Verification items for the finished model (mm, model axes). Coordinates: 2 decimals unless noted, no trailing zeros. Order: outer loops, then holes, each group sorted by start corner. A loop starts at its lowest first (then second) coordinate and runs counter-clockwise, first axis right, second up. Notation, with made-up numbers: (89.25, 8) - (143.25, 8) arc R6 ccw to (143.25, 15) - close; hole circle Ø9 at (31, 63). An arc over 180 degrees is marked (long way). One line per question, with ' | ' between items. Start each with the question number.
from build123d import *

# Parameters (mm, degrees)
F0_R     = 3.3
F0_R_2   = 4.5
F1_DEPTH = 1
F2_D     = 6.6
F3_D     = 6.6
F4_D     = 9


with BuildPart() as f1:
    # F0 (on Top) → F1 (new body)
    with BuildSketch(Plane.XY):
        with Locations((0, 16)):
            Circle(F0_R)
        Circle(F0_R_2)
        with Locations((0, -16)):
            Circle(F0_R)
        with BuildLine():
            ThreePointArc((0, 10), (6.123724, 7.905694), (9.682458, 2.5))
            Line((9.682458, 2.5), (5.809475, 17.5))
            ThreePointArc((5.809475, 17.5), (5.952178, 16.756026), (6, 16))
            ThreePointArc((6, 16), (4.242641, 11.757359), (0, 10))
        make_face()
        with BuildLine():
            ThreePointArc((-9.682458, 2.5), (-6.123724, 7.905694), (0, 10))
            ThreePointArc((0, 10), (-4.743416, 12.325765), (-5.809475, 17.5))
            Line((-5.809475, 17.5), (-9.682458, 2.5))
        make_face()
        with BuildLine():
            Line((5.809475, -17.5), (9.682458, -2.5))
            ThreePointArc((9.682458, -2.5), (6.123724, -7.905694), (0, -10))
            ThreePointArc((0, -10), (4.242641, -11.757359), (6, -16))
            ThreePointArc((6, -16), (5.952178, -16.756026), (5.809475, -17.5))
        make_face()
        with BuildLine():
            ThreePointArc((-5.809475, -17.5), (-4.743416, -12.325765), (0, -10))
            ThreePointArc((0, -10), (-6.123724, -7.905694), (-9.682458, -2.5))
            Line((-9.682458, -2.5), (-5.809475, -17.5))
        make_face()
        with BuildLine():
            ThreePointArc((6, -16), (4.242641, -11.757359), (0, -10))
            ThreePointArc((0, -10), (-4.743416, -12.325765), (-5.809475, -17.5))
            ThreePointArc((-5.809475, -17.5), (0, -22), (5.809475, -17.5))
            ThreePointArc((5.809475, -17.5), (5.952178, -16.756026), (6, -16))
        make_face()
        with Locations((0, -16)):
            Circle(F0_R, mode=Mode.SUBTRACT)
        with BuildLine():
            ThreePointArc((-5.809475, 17.5), (-4.743416, 12.325765), (0, 10))
            ThreePointArc((0, 10), (4.242641, 11.757359), (6, 16))
            ThreePointArc((6, 16), (5.952178, 16.756026), (5.809475, 17.5))
            ThreePointArc((5.809475, 17.5), (0, 22), (-5.809475, 17.5))
        make_face()
        with Locations((0, 16)):
            Circle(F0_R, mode=Mode.SUBTRACT)
        with BuildLine():
            ThreePointArc((9.682458, -2.5), (9.920297, -1.260043), (10, 0))
            ThreePointArc((10, 0), (9.920297, 1.260043), (9.682458, 2.5))
            ThreePointArc((9.682458, 2.5), (6.123724, 7.905694), (0, 10))
            ThreePointArc((0, 10), (-6.123724, 7.905694), (-9.682458, 2.5))
            ThreePointArc((-9.682458, 2.5), (-10, 0), (-9.682458, -2.5))
            ThreePointArc((-9.682458, -2.5), (-6.123724, -7.905694), (0, -10))
            ThreePointArc((0, -10), (6.123724, -7.905694), (9.682458, -2.5))
        make_face()
        Circle(F0_R_2, mode=Mode.SUBTRACT)
    extrude(amount=F1_DEPTH)

    # F2 (through all)
    with Locations(Plane(origin=(0, 0, 0), x_dir=(1, 0, 0), z_dir=(0, 0, -1))):
        with Locations((0, 16)):
            Hole(F2_D / 2)

    # F3 (through all)
    with Locations(Plane(origin=(0, 0, 0), x_dir=(1, 0, 0), z_dir=(0, 0, -1))):
        with Locations((0, -16)):
            Hole(F3_D / 2)

    # F4 (through all)
    with Locations(Plane(origin=(0, 0, 0), x_dir=(1, 0, 0), z_dir=(0, 0, -1))):
        with Locations((0, 0)):
            Hole(F4_D / 2)


solid = f1.part
Item 1: Section check D-D (x = 4). Record the cut outline in (y, z).
Item 2: Section check B-B (x = 0). Record the cut outline in (y, z).
Item 3: Section check A-A (z = 0.3). Record the cut outline in (x, y).
Item 4: Mould release check, pull along X, two halves, no side actions. Record for faces 1 (the flat face through (7.72, -10.1, 0.49)), 2 (the cylindrical face through (-10, 0, 0.5)), 3 (the cylindrical face through (-2.619, -18.008, 0.493)), 4 (the cylindrical face through (-2.43, 18.23, 0.49)): +X half, -X half, draft (parallel to the pull), parting line (faces both ways), or undercut.
Item 5: Thickness scan on probe 1 along Y at (x, z) = (1.5, 0.2); probe 2 along Y at (x, z) = (-2, 0.8); probe 3 along X at (y, z) = (-1, 0.7). Record the ranges inside material, lowest first. Write a range as from..to.
Item 6: Gauge pin test, flat end, axial feed: pin 1 (2 mm diameter, centred on x = 0, y = 2, fed in from -Z). Record the tip position at first contact, or that the pin passes through.
Item 7: Section check C-C (y = -16). Record the cut outline in (x, z).
Completed:
1) outline: (-20.47, 0) - (-2.06, 0) - (-2.06, 1) - (-20.47, 1) - close; (2.06, 0) - (20.47, 0) - (20.47, 1) - (2.06, 1) - close
2) outline: (-22, 0) - (-19.3, 0) - (-19.3, 1) - (-22, 1) - close; (-12.7, 0) - (-4.5, 0) - (-4.5, 1) - (-12.7, 1) - close; (4.5, 0) - (12.7, 0) - (12.7, 1) - (4.5, 1) - close; (19.3, 0) - (22, 0) - (22, 1) - (19.3, 1) - close
3) outline: (-9.68, -2.5) - (-5.81, -17.5) arc R6 ccw to (5.81, -17.5) - (9.68, -2.5) arc R10 ccw to (10, 0) arc R10 ccw to (9.68, 2.5) - (5.81, 17.5) arc R6 ccw to (-5.81, 17.5) - (-9.68, 2.5) arc R10 ccw to start; hole circle Ø9 at (0, 0); hole circle Ø6.6 at (0, -16); hole circle Ø6.6 at (0, 16)
4) face 1: +X half | face 2: -X half | face 3: undercut | face 4: undercut
5) probe 1: y = -21.81..-18.94, -13.06..-4.24, 4.24..13.06, 18.94..21.81 | probe 2: y = -21.66..-18.62, -13.38..-4.03, 4.03..13.38, 18.62..21.66 | probe 3: x = -9.95..-4.39, 4.39..9.95
6) pin 1: passes through
7) outline: (-6.2, 0) - (-3.3, 0) - (-3.3, 1) - (-6.2, 1) - close; (3.3, 0) - (6.2, 0) - (6.2, 1) - (3.3, 1) - close
